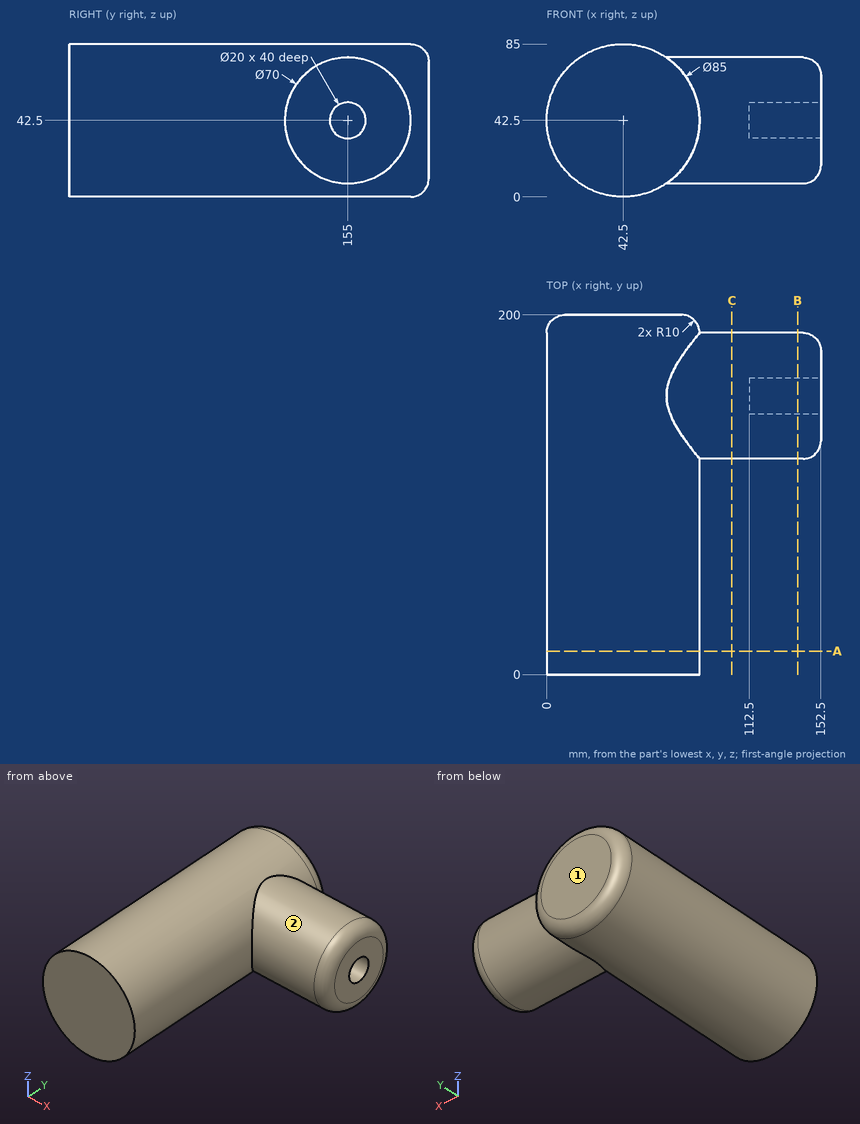
Design review of the part shown in the three views and the two pictorial views. Dimensions are in mm from the part's minimum x, y and z. A direction names the side the tool comes from. Give positions to 0.01 mm unless a question says otherwise; leave off trailing zeros. Loops run counter-clockwise (first coordinate to the right, second up) from the corner with the lowest first, then second, coordinate; pieces in that order, holes last. Notation, with made-up numbers: (38.5, 16) -> (65.5, 16) arc R23 ccw to (65.5, 49) -> close; hole circle Ø6 at (-34, -9.5). An arc over 180 degrees is marked (long way). One line per item, written item: value.
Q1. Machinability: for the marked faces 1 and 2, which of the approach directions +Z, -Z, +X, -X, +Y, -Y give a long, thin tool a straight path to every point of the face, cutting with its end or side? Answer none if there is none.
Numbers:
face 1: +Z, -Z, +X, -X, +Y
face 2: +X
Q2. We need section B-B on x = 139.5. Give the boundary of the cut face in (y, z).
Numbers:
outline: circle Ø70 at (155, 42.5); hole circle Ø20 at (155, 42.5)
Q3. We need section C-C on x = 103. Give the boundary of the cut face in (y, z).
Numbers:
outline: circle Ø70 at (155, 42.5)
Q4. For pin 1 Ø6 at (y, z) = (157.5, 41.5) entering from +X; pin 2 Ø6 at (y, z) = (160, 67.5) entering from -X; pin 3 Ø3 at (x, y) = (110.5, 154.5) entering from +Z, all flat-tipped, find the tip position at first contact; note any pin that passes through.
Numbers:
pin 1: stops at x = 112.5
pin 2: stops at x = 6.14
pin 3: stops at z = 77.5
Q5. We need section A-A on y = 13. Give the boundary of the cut face in (x, z).
Numbers:
outline: circle Ø85 at (42.5, 42.5)
Q6. For L1, parallel to Y at x = 134, z = 42.5; L2, parallel to Z at x = 120, y = 156; L3, parallel to X at y = 20.5, z = 44, list the stretches that pass through material, from the lowest coordinate up.
Numbers:
L1: y = 120 to 145, 165 to 190
L2: z = 7.51 to 32.55, 52.45 to 77.49
L3: x = 0.03 to 84.97
